Autodesk Inventor part; units mm, degrees
ref_plane "YZ Plane" through (0, 0, 0) normal (1, 0, 0) x (0, 1, 0)
ref_plane "XZ Plane" through (0, 0, 0) normal (0, 1, 0) x (-1, 0, 0)
ref_plane "XY Plane" through (0, 0, 0) normal (0, 0, 1) x (1, 0, 0)
sketch "Sketch1" plane through (0, 0, 0) normal (0, 0, 1) x (1, 0, 0)
  line L0 (0, 0) -> (19.5, 0)
  line L1 (19.5, 0) -> (19.5, 29.5)
  line L2 (19.5, 29.5) -> (0, 29.5)
  line L3 (0, 29.5) -> (0, 0)
  dimension "d0" = 19.5
  dimension "d1" = 29.5
extrude "Extrusion1" add sketch "Sketch1" along normal blind 40
sketch "Sketch2" plane through (0, 0, 0) normal (0, -1, 0) x (1, 0, 0)
  line L0 (0, 0) -> (19.5, 0)
  line L1 (9.75, 0) -> (9.75, 2.5)
  line L2 (9.75, 2.5) -> (14.75, 2.5)
  line L3 (14.75, 2.5) -> (4.75, 2.5)
  circle A0 centre (4.75, 2.5) radius 2.75
  circle A1 centre (14.75, 2.5) radius 2.75
  dimension "d4" = 2.5
  dimension "d5" = 5
  dimension "d6" = 10
  dimension "d7" = 5.5
  dimension "d8" = 5.5
extrude "Extrusion2" cut sketch "Sketch2" against normal through all contours A0 L0 | L0 A0 | A1 L0 | L0 A1
sketch "Sketch3" plane through (0, 0, 0) normal (0, 0, -1) x (-1, 0, 0)
  line L0 (0, 29.5) -> (0, 0)
  line L1 (0, 14.75) -> (-19.5, 14.75)
  line L2 (-19.5, 0) -> (-19.5, 29.5)
  line L3 (-19.5, 14.75) -> (-19.5, 12.75)
  line L4 (-19.5, 12.75) -> (-19.5, 16.75)
  line L5 (-19.5, 16.75) -> (0, 16.75)
  line L6 (0, 16.75) -> (0, 12.75)
  line L7 (0, 12.75) -> (-19.5, 12.75)
  dimension "d11" = 2
  dimension "d12" = 4
extrude "Extrusion3" cut sketch "Sketch3" against normal blind 9
sketch "Sketch4" plane through (0, 0, 40) normal (0, -1, 0) x (1, 0, 0)
  line L0 (19.5, 0) -> (0, 0)
  line L1 (9.75, 0) -> (9.75, -17.5)
  line L2 (9.75, -17.5) -> (9.75, -10)
  circle A0 centre (9.75, -10) radius 1.375
  circle A1 centre (9.75, -6.75) radius 1.375
  circle A2 centre (9.75, -3.5) radius 1.375
  circle A3 centre (9.75, -0.25) radius 1.375
  circle A4 centre (2.25, -17.5) radius 1.375
  circle A5 centre (-1, -17.5) radius 1.375
  circle A6 centre (-4.25, -17.5) radius 1.375
  circle A7 centre (-7.5, -17.5) radius 1.375
  circle A8 centre (9.75, -25) radius 1.375
  circle A9 centre (9.75, -28.25) radius 1.375
  circle A10 centre (9.75, -31.5) radius 1.375
  circle A11 centre (9.75, -34.75) radius 1.375
  circle A12 centre (17.25, -17.5) radius 1.375
  circle A13 centre (20.5, -17.5) radius 1.375
  circle A14 centre (23.75, -17.5) radius 1.375
  circle A15 centre (27, -17.5) radius 1.375
  point P0 (0, -40)
  dimension "d15" = 17.5
  dimension "d16" = 7.5
  dimension "d17" = 2.75
  dimension "d20" = 3.25
  dimension "d27" = 360
extrude "Extrusion4" cut sketch "Sketch4" against normal through all
properties part number "wirst fix"
Read the model definition and answer for the solid it produces. Units are mm, in the model's axes. Round coordinates to 2 decimals unless told otherwise and drop trailing zeros. Loops run counter-clockwise (first coordinate to the right, second up) from the corner with the lowest first, then second, coordinate; pieces in that order, holes last.
Q1. Section D-D on y = 14.5 is taken. Write down the section's boundary in (x, z) (3 decimals).
Q2. Consider probe 1 along X at (y, z) = (24.75, 2.5); probe 2 along X at (y, z) = (17.75, 33.25) (3 decimals); probe 3 along Z at (x, y) = (9.75, 14.25) (3 decimals). Determine where each line is inside the solid, lowest interval first.
Q3. This flat-tipped pin is pushed along its axis until it touches: pin 1 (1.6 mm diameter, centred on x = 9.75, z = 5.25, fed in from +Y). Where does it stop, or does it pass through?
Q4. Section A-A on z = 22.5 is taken. Write down the section's boundary in (x, y) (3 decimals).
Q5. Section B-B on x = 14.75 is taken. Write down the section's boundary in (y, z), and give its area (3 significant figures).
Q6. Determine the mould class of faces 1 (the face through (10, 12.75, 3)), 2 (the face through (10, 29.5, 20)), 3 (the face through (15, 15, 9)), 4 (the face through (9.716, 14.544, 38.375)) for opening direction Y: released by +Y, released by -Y, zero draft, split by the parting line, or undercut.
Q7. Section C-C on z = 11.75 is taken. Write down the section's boundary in (x, y) (3 decimals).
Output:
1. outline: (0, 9) - (8.469, 9) arc R1.375 cw to (11.031, 9) - (19.5, 9) - (19.5, 21.556) arc R1.375 cw to (19.5, 23.444) - (19.5, 40) - (11.102, 40) arc R1.375 cw (long way) to (8.398, 40) - (0, 40) - (0, 23.444) arc R1.375 cw to (0, 21.556) - close; hole circle Ø2.75 at (2.25, 22.5); hole circle Ø2.75 at (9.75, 11.75); hole circle Ø2.75 at (9.75, 15); hole circle Ø2.75 at (9.75, 30); hole circle Ø2.75 at (9.75, 33.25); hole circle Ø2.75 at (9.75, 36.5); hole circle Ø2.75 at (17.25, 22.5)
2. probe 1: x = 0 to 2, 7.5 to 12, 17.5 to 19.5
2. probe 2: x = 0 to 8.375, 11.125 to 19.5
2. probe 3: z = 9.875 to 10.375, 13.125 to 13.625, 16.375 to 28.625, 31.375 to 31.875, 34.625 to 35.125, 37.875 to 38.375
3. pin 1: passes through
4. outline: (0.375, 0) - (0.875, 0) - (0.875, 29.5) - (0.375, 29.5) - close; (3.625, 0) - (15.875, 0) - (15.875, 29.5) - (3.625, 29.5) - close; (18.625, 0) - (19.125, 0) - (19.125, 29.5) - (18.625, 29.5) - close
5. outline: (0, 5.25) - (12.75, 5.25) - (12.75, 9) - (16.75, 9) - (16.75, 5.25) - (29.5, 5.25) - (29.5, 40) - (0, 40) - close
5. area: 1,010 mm2
6. face 1: undercut
6. face 2: released by +Y
6. face 3: undercut
6. face 4: zero draft
7. outline: (0, 0) - (8.375, 0) - (8.375, 29.5) - (0, 29.5) - close; (11.125, 0) - (19.5, 0) - (19.5, 29.5) - (11.125, 29.5) - close
